CAD build for the part. Positions are in the model's coordinates, mm. A direction names the side the tool comes from. Round coordinates to 2 decimals unless told otherwise and drop trailing zeros. Write each loop counter-clockwise with the first axis right and the second up, starting at its lowest first coordinate (ties: lowest second). Pieces come first, ordered by that corner, then holes. Notation, with made-up numbers: (73.5, -18) -> (100.5, -18) arc R18 ccw to (100.5, 14) -> close; hole circle Ø8 at (-21.5, 21). An arc over 180 degrees is marked (long way). Put each result on its own line as item: value. Start each with the question number.
1. Saw through at A-A on x = 29. List the corners of the cut face in (y, z).
2. Pull direction Y, two halves, no side cores. Call faces 1 (the flat face through (63.48, 14.924, 12.325)), 2 (the cylindrical face through (-1.172, 8.923, 12.675)), 3 (the flat face through (-75, 10, 12)): pulls with the +Y half, pulls with the -Y half, needs draft (parallel to the pull), parting line crosses it, or undercut.
3. 3-axis set-ups, long thin cutter, end or side, ignore diameter. For faces 4 (the flat face through (46, -7.459, 12)), 5 (the flat face through (-46, -7.459, 12)), 6 (the flat face through (-2, -17.459, 12)): which of +Z, -Z, +X, -X, +Y, -Y reach the whole face in a straight line?
4. Saw through at C-C on z = 14.5. List the corners of the cut face in (x, y), and give its area (3 significant figures).
5. Saw through at B-B on y = 0. List the corners of the cut face in (x, z), and give its area (3 significant figures).
6. Flat gauge pins, fed straight in: P1, Ø10, axis at y = -6, z = 5.5, coming from the -X side; P2, Ø3.5, axis at y = 0.5, z = 10.5, coming from the -X side; P3, Ø7.5, axis at x = 56.5, z = 9.5, coming from the -Y side; P4, Ø8.5, axis at y = -2, z = 18.5, coming from the +X side. Where does each tip first touch, or does it go through?
7. Drill centre lines: line 1 (Y direction, x = 0, z = 11.25); line 2 (X direction, y = 0.5, z = 2.5); line 3 (X direction, y = -1, z = 11.25). Where is each one in solid material? Low to high. Write a range as from..to.
from build123d import *

# Parameters (mm, degrees)
F1_DEPTH = 25
F2_R     = 9
F3_DEPTH = 40
F4_R     = 2


with BuildPart() as f1:
    # F0 (on Top) → F1 (new body)
    with BuildSketch(Plane.XY):
        Polygon((-15, -7.459), (-75, -7.459), (-75, -12.459), (-54.951493, -17.459), (51.843371, -17.459), (75, -12.459), (75, -7.459), (15, -7.459), (15, 7.459), (75, 7.459), (75, 12.459), (51.631901, 17.459), (-54.528542, 17.459), (-75, 12.459), (-75, 7.459), (-15, 7.459), align=None)
    extrude(amount=F1_DEPTH)

    # F2 (on face) → F3 (cut)
    with BuildSketch(Plane.XY.offset(25)):
        Circle(F2_R)
    extrude(amount=-F3_DEPTH, mode=Mode.SUBTRACT)

    # F4
    f4_edges = [f1.edges().sort_by_distance(p)[0] for p in [
        (-15, -7.459, 12.5),
        (-15, 7.459, 12.5),
        (15, -7.459, 12.5),
        (15, 7.459, 12.5),
    ]]
    fillet(f4_edges, radius=F4_R)


solid = f1.part
Return value:
1. outline: (-17.46, 0) -> (-7.46, 0) -> (-7.46, 25) -> (-17.46, 25) -> close; (7.46, 0) -> (17.46, 0) -> (17.46, 25) -> (7.46, 25) -> close
2. face 1: pulls with the +Y half
2. face 2: undercut
2. face 3: needs draft
3. face 4: +Z, -Z, +X
3. face 5: +Z, -Z, -X
3. face 6: +Z, -Z, +X, -X, -Y
4. outline: (-75, -12.46) -> (-54.95, -17.46) -> (51.84, -17.46) -> (75, -12.46) -> (75, -7.46) -> (17, -7.46) arc R2 cw to (15, -5.46) -> (15, 5.46) arc R2 cw to (17, 7.46) -> (75, 7.46) -> (75, 12.46) -> (51.63, 17.46) -> (-54.53, 17.46) -> (-75, 12.46) -> (-75, 7.46) -> (-17, 7.46) arc R2 cw to (-15, 5.46) -> (-15, -5.46) arc R2 cw to (-17, -7.46) -> (-75, -7.46) -> close; hole circle Ø18 at (0, 0)
4. area: 2,980 mm^2
5. outline: (-15, 0) -> (-9, 0) -> (-9, 25) -> (-15, 25) -> close; (9, 0) -> (15, 0) -> (15, 25) -> (9, 25) -> close
5. area: 300 mm^2
6. P1: stops at x = -75
6. P2: stops at x = -15
6. P3: stops at y = -17.26
6. P4: stops at x = 15.16
7. line 1: y = -17.46..-9, 9..17.46
7. line 2: x = -15..-8.99, 8.99..15
7. line 3: x = -15..-8.94, 8.94..15
